For this review, take the finished solid that the model builds, in its own axes (mm). Give positions to 0.01 mm unless a question says otherwise; leave off trailing zeros. Loops run counter-clockwise (first coordinate to the right, second up) from the corner with the lowest first, then second, coordinate; pieces in that order, holes last. Notation, with made-up numbers: (-39.5, 16.25) - (18.5, 16.25) arc R32 ccw to (18.5, 45.25) - close; hole circle Ø3 at (-36.5, 66). An arc over 180 degrees is marked (long way). Answer as CSV lines item,"result".
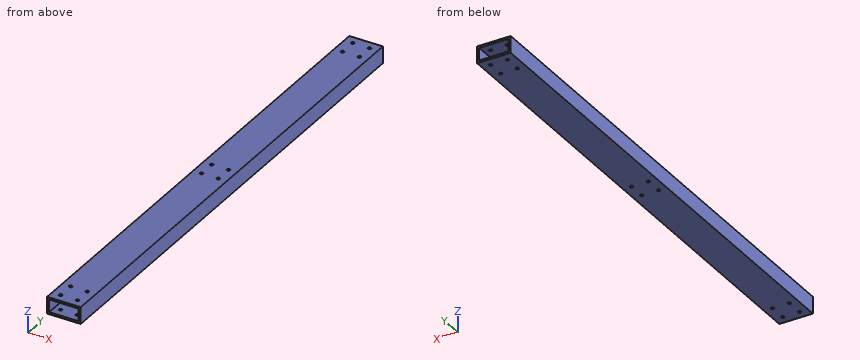
from build123d import *

# Parameters (mm, degrees)
SKETCH1_W               = 50.8
SKETCH1_H               = 25.4
BOSS_EXTRUDE1_DEPTH     = 381
SHELL1_T                = -3.175
CUT_EXTRUDE2_DEPTH      = 383.689587002
CUT_EXTRUDE2_DEPTH_BACK = 383.689587002
SKETCH5_R               = 2.38125


with BuildPart() as part:
    # Sketch1 → Boss-Extrude1 (new, symmetric)
    with BuildSketch(Plane(origin=(0, 0, 0), x_dir=(1, 0, 0), z_dir=(0, 1, 0))):
        Rectangle(SKETCH1_W, SKETCH1_H)
    extrude(amount=BOSS_EXTRUDE1_DEPTH, both=True)

    # Shell1
    shell1_openings = [part.faces().sort_by_distance(p)[0] for p in [
        (0, 381, 0),
        (0, -381, 0),
    ]]
    offset(amount=SHELL1_T, openings=shell1_openings, kind=Kind.INTERSECTION)

    # Sketch5 → Cut-Extrude2 (cut, two sides: drawn at the far end of the back side and taken through both)
    with BuildSketch(Plane.XY.offset(12.7).offset(-CUT_EXTRUDE2_DEPTH_BACK)):
        with Locations((-12.7, 368.3)):
            Circle(SKETCH5_R)
        with Locations((12.7, 368.3)):
            Circle(SKETCH5_R)
        with Locations((12.7, 342.9)):
            Circle(SKETCH5_R)
        with Locations((-12.7, 342.9)):
            Circle(SKETCH5_R)
        with Locations((-12.7, -342.9)):
            Circle(SKETCH5_R)
        with Locations((12.7, -342.9)):
            Circle(SKETCH5_R)
        with Locations((12.7, -368.3)):
            Circle(SKETCH5_R)
        with Locations((-12.7, -368.3)):
            Circle(SKETCH5_R)
        with Locations((-12.7, 12.7)):
            Circle(SKETCH5_R)
        with Locations((12.7, 12.7)):
            Circle(SKETCH5_R)
        with Locations((12.7, -12.7)):
            Circle(SKETCH5_R)
        with Locations((-12.7, -12.7)):
            Circle(SKETCH5_R)
    extrude(amount=CUT_EXTRUDE2_DEPTH + CUT_EXTRUDE2_DEPTH_BACK, mode=Mode.SUBTRACT)


solid = part.part
1) Wall thickness on line 1 (X direction, y = 12.7, z = 11.7); line 2 (X direction, y = -141, z = 5.5) (3 decimals); line 3 (Z direction, x = 18.5, y = -166) (3 decimals): over which ranges is each line inside the solid? List them lowest first. Write a range as from..to.
From the geometry:
line 1,"x = -25.4..-15.08, -10.32..10.32, 15.08..25.4"
line 2,"x = -25.4..-22.225, 22.225..25.4"
line 3,"z = -12.7..-9.525, 9.525..12.7"
2) Consider section A-A on x = -3. Write out the cut boundary in (y, z) (3 decimals).
From the geometry:
outline,"(-381, -12.7) - (381, -12.7) - (381, -9.525) - (-381, -9.525) - close; (-381, 9.525) - (381, 9.525) - (381, 12.7) - (-381, 12.7) - close"
3) Consider section B-B on z = 3.5. Write out the cut boundary in (x, y) (3 decimals).
From the geometry:
outline,"(-25.4, -381) - (-22.225, -381) - (-22.225, 381) - (-25.4, 381) - close; (22.225, -381) - (25.4, -381) - (25.4, 381) - (22.225, 381) - close"
4) Consider section C-C on y = -260. Write out the cut boundary in (x, z) (3 decimals), and give its area (3 significant figures).
From the geometry:
outline,"(-25.4, -12.7) - (25.4, -12.7) - (25.4, 12.7) - (-25.4, 12.7) - close; hole (-22.225, -9.525) - (22.225, -9.525) - (22.225, 9.525) - (-22.225, 9.525) - close"
area,"444 mm^2"
5) Insertion check: P1, Ø4, axis at x = -12.7, y = -12.7, coming from the +Z side. The pin has a flat end and moves straight along its axis. Give the tip position at first contact, or say it passes through.
From the geometry:
P1,"passes through"
